Source: three-view drawing plus pictorial views. Frame: mm from the lowest corner of the part. Coordinates: 2 decimals unless noted, no trailing zeros. Order: outer loops, then holes, each group sorted by start corner. A loop starts at its lowest first (then second) coordinate and runs counter-clockwise, first axis right, second up. Notation, with made-up numbers: (39.5, 40.25) -> (53.5, 40.25) arc R11 ccw to (53.5, 54.25) -> close; hole circle Ø11 at (58.5, 73). An arc over 180 degrees is marked (long way). Use one line per item in the form item = value. Start each with the question number.
1) Section query C-C on z = 2.5. Output: boundary loops of the cut face in (x, y) (1 decimal).
2) Pin query (flat end, axial travel): pin 1 (3.5 mm diameter, centred on x = 95.8, y = 66.5, fed in from +Z) (1 decimal); pin 2 (3 mm diameter, centred on x = 255, y = 39.5, fed in from -Z) (1 decimal); pin 3 (6 mm diameter, centred on x = 419, y = 66.5, fed in from -Z). Return the tip coordinate at first contact, or that it passes through.
3) Section query A-A on x = 139.5. Output: boundary loops of the cut face in (y, z) (1 decimal).
4) Ray query, line 1 along Z through (x, y) = (182.5, 126) (1 decimal); line 2 along Z through (x, y) = (38.5, 28) (1 decimal). Return the intervals inside material, ascending.
5) Section query B-B on y = 23. Output: boundary loops of the cut face in (x, z) (1 decimal), then the cut area to 3 significant figures.
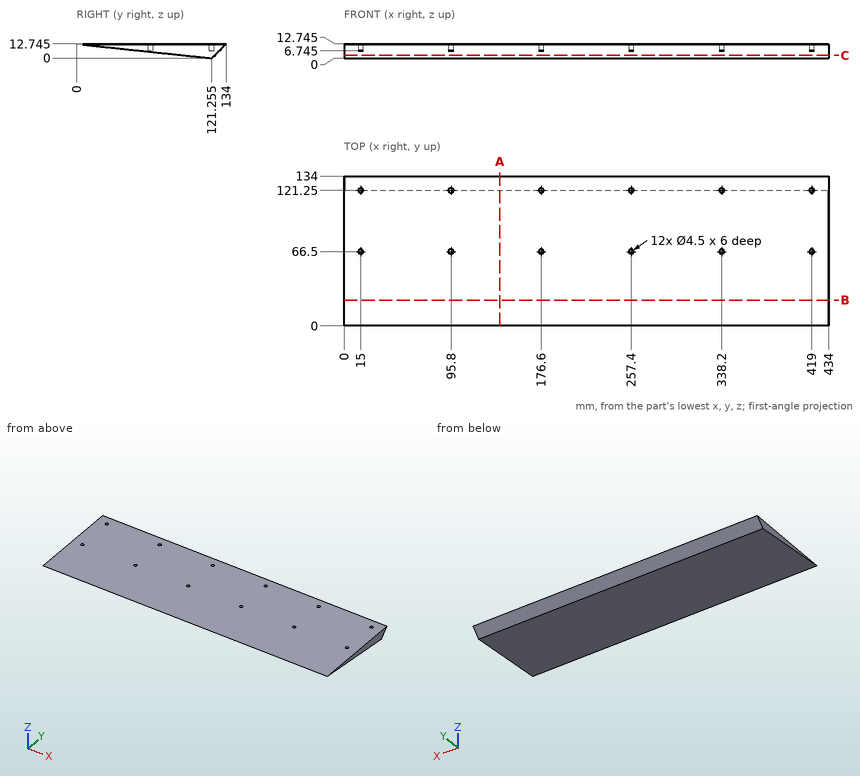
Answers below:
q1.outline = (0, 97.5) -> (434, 97.5) -> (434, 123.8) -> (0, 123.8) -> close
q2.pin_1 = 6.7
q2.pin_2 = 8.4
q2.pin_3 = 5.44
q3.outline = (0, 12.7) -> (121.3, 0) -> (134, 12.7) -> close
q4.line_1 = 4.7 to 12.7
q4.line_2 = 9.8 to 12.7
q5.outline = (0, 10.3) -> (434, 10.3) -> (434, 12.7) -> (0, 12.7) -> close
q5.area = 1,050 mm^2
